Can you work these out from the model? Positions are in its coordinate system, mm. A direction names the side the tool comes from. Give positions to 0.01 mm unless a question says otherwise; leave off trailing zeros. Loops run counter-clockwise (first coordinate to the right, second up) from the corner with the lowest first, then second, coordinate; pieces in that order, holes last. Notation, with made-up numbers: (84.5, 41.5) - (114.5, 41.5) arc R10 cw to (114.5, 51.5) - close; hole circle Ø11 at (35.5, 1). An arc over 180 degrees is marked (long way). Answer as a JSON object with one key per item and string values. Group by question number.
Item 1: Suppose I cut it at B-B on y = 3.1. Write out the boundary of the cut face in (x, z), and give its area (3 significant figures).
Item 2: Suppose I cut it at A-A on z = 0. Write out the boundary of the cut face in (x, y), and give its area (4 significant figures).
Item 3: Thinking about a two-plate mould opening in X: for faces 1 (the cylindrical face through (-47.26, 3.52, 3.75)), 2 (the cylindrical face through (-31.21, 3.52, 0.04)), 3 (the cylindrical face through (15, 2, 0)), 4 (the flat face through (-25, 2, 15)), which applies, pulls with the +X half, pulls with the -X half, needs draft (parallel to the pull), parting line crosses it, or undercut?
Item 4: Suppose I cut it at D-D on z = 8. Write out the boundary of the cut face in (x, y).
Item 5: Which directions (+Z, -Z, +X, -X, +Y, -Y) give clear straight access to the entire face, cutting with the end or side of a thin tool? Please do faces 5 (the flat face through (-24, 0, 0)), 6 (the flat face through (-47, 2, -3)).
Item 6: Suppose I cut it at C-C on z = -9. Write out the boundary of the cut face in (x, y), and give its area (3 significant figures).
Item 7: Please list where these lines run through material, in increasing order: L1, parallel to X at y = 0.4, z = 0; L2, parallel to X at y = 3.4, z = 0; L3, parallel to Z at x = -0.5, y = 0.65.
Item 8: Will these pins go through, and if not, where does the flat tip stop? pin 1 (6 mm diameter, centred on x = -47.21, z = 0, fed in from +Y); pin 2 (1.5 mm diameter, centred on y = 3, z = -8, fed in from +X).
from build123d import *

# Parameters (mm, degrees)
RESSALTO_EXTRUS_O2_DEPTH = 5
ESBO_O4_R                = 1.75
CORTE_EXTRUS_O1_DEPTH    = 10
CORTE_EXTRUS_O2_DEPTH    = 3
ESBO_O7_R                = 2.5
CORTE_EXTRUS_O3_DEPTH    = 67.895440801


with BuildPart() as part:
    # Esboço3 → Ressalto-extrusão2 (new body)
    with BuildSketch(Plane(origin=(0, 0, 0), x_dir=(1, 0, 0), z_dir=(0, 1, 0))):
        with BuildLine():
            Line((-50, 15), (0, 15))
            ThreePointArc((0, 15), (15, 0), (0, -15))
            Line((0, -15), (-50, -15))
            ThreePointArc((-50, -15), (-65, 0), (-50, 15))
        make_face()
    extrude(amount=RESSALTO_EXTRUS_O2_DEPTH)

    # Esboço4 → Corte-extrusão1 (cut)
    with BuildSketch(Plane(origin=(0, 5, 0), x_dir=(1, 0, 0), z_dir=(0, 1, 0))):
        with Locations(Location((0, 0, 0), (0, 0, 90))):
            Circle(ESBO_O4_R)
    extrude(amount=-CORTE_EXTRUS_O1_DEPTH, mode=Mode.SUBTRACT)

    # Esboço6 → Corte-extrusão2 (cut)
    with BuildSketch(Plane(origin=(0, 5, 0), x_dir=(1, 0, 0), z_dir=(0, 1, 0))):
        with BuildLine():
            Line((-50.096108497, 2.395111434), (-61.281465627, 1.998745461))
            ThreePointArc((-61.281465627, 1.998745461), (-63.210637787, 0), (-61.281465627, -1.998745461))
            Line((-61.281465627, -1.998745461), (-50.096108497, -2.395111434))
            ThreePointArc((-50.096108497, -2.395111434), (-47.210637787, -3.75), (-44.325167077, -2.395111434))
            Line((-44.325167077, -2.395111434), (-33.139809947, -1.998745461))
            ThreePointArc((-33.139809947, -1.998745461), (-31.210637787, 0), (-33.139809947, 1.998745461))
            Line((-33.139809947, 1.998745461), (-44.325167077, 2.395111434))
            ThreePointArc((-44.325167077, 2.395111434), (-47.210637787, 3.75), (-50.096108497, 2.395111434))
        make_face()
        with BuildLine():
            ThreePointArc((-47.443873787, 2.489096416), (-47.210637787, 2.5), (-46.977401787, 2.489096416))
            ThreePointArc((-46.977401787, 2.489096416), (-45.362247947, 1.683286963), (-44.710637787, 0))
            ThreePointArc((-44.710637787, 0), (-45.362247947, -1.683286963), (-46.977401787, -2.489096416))
            ThreePointArc((-46.977401787, -2.489096416), (-47.210637787, -2.5), (-47.443873787, -2.489096416))
            ThreePointArc((-47.443873787, -2.489096416), (-49.710637787, 0), (-47.443873787, 2.489096416))
        make_face(mode=Mode.SUBTRACT)
    extrude(amount=-CORTE_EXTRUS_O2_DEPTH, mode=Mode.SUBTRACT)

    # Esboço7 → Corte-extrusão3 (cut, through all)
    with BuildSketch(Plane(origin=(0, 5, 0), x_dir=(1, 0, 0), z_dir=(0, 1, 0))):
        with Locations(Location((-47.210637787, 0, 0), (0, 0, 270))):
            Circle(ESBO_O7_R)
    extrude(amount=-CORTE_EXTRUS_O3_DEPTH, mode=Mode.SUBTRACT)


solid = part.part
Worked out:
{
 "1": {"outline": "(-50, -15) - (0, -15) arc R15 ccw to (0, 15) - (-50, 15) arc R15 ccw to start; hole (-61.28, -2) - (-50.1, -2.4) arc R3.75 ccw to (-44.33, -2.4) - (-33.14, -2) arc R2 ccw to (-33.14, 2) - (-44.33, 2.4) arc R3.75 ccw to (-50.1, 2.4) - (-61.28, 2) arc R2 ccw to start; hole circle Ø3.5 at (0, 0)", "area": "2,050 mm2"},
 "2": {"outline": "(-65, 0) - (-49.71, 0) - (-49.71, 2) - (-63.21, 2) - (-63.21, 5) - (-65, 5) - close; (-44.71, 0) - (-1.75, 0) - (-1.75, 5) - (-31.21, 5) - (-31.21, 2) - (-44.71, 2) - close; (1.75, 0) - (15, 0) - (15, 5) - (1.75, 5) - close", "area": "276.5 mm2"},
 "3": {"face 1": "undercut", "face 2": "undercut", "face 3": "pulls with the +X half", "face 4": "needs draft"},
 "4": {"outline": "(-62.69, 0) - (12.69, 0) - (12.69, 5) - (-62.69, 5) - close"},
 "5": {"face 5": "+Z, -Z, +X, -X, -Y", "face 6": "+Y"},
 "6": {"outline": "(-62, 0) - (12, 0) - (12, 5) - (-62, 5) - close", "area": "370 mm2"},
 "7": {"L1": "x = -65 to -49.71, -44.71 to -1.75, 1.75 to 15", "L2": "x = -65 to -63.21, -31.21 to -1.75, 1.75 to 15", "L3": "z = -15 to -1.68, 1.68 to 15"},
 "8": {"pin 1": "stops at y = 2", "pin 2": "stops at x = 13.13"}
}
